The drawing under review shows one solid part. Ordinate dimensions are in mm from its lowest x, y, z. Coordinates: 2 decimals unless noted, no trailing zeros. Loops run counter-clockwise (first coordinate to the right, second up) from the corner with the lowest first, then second, coordinate; pieces in that order, holes last. Notation, with made-up numbers: M 69.5,-16 L 97.5,-16 A30 ccw 97.5,6 Z; hole C -26.5,83 d3. An arc over 180 degrees is marked long. Use one line per item in the form item = value.
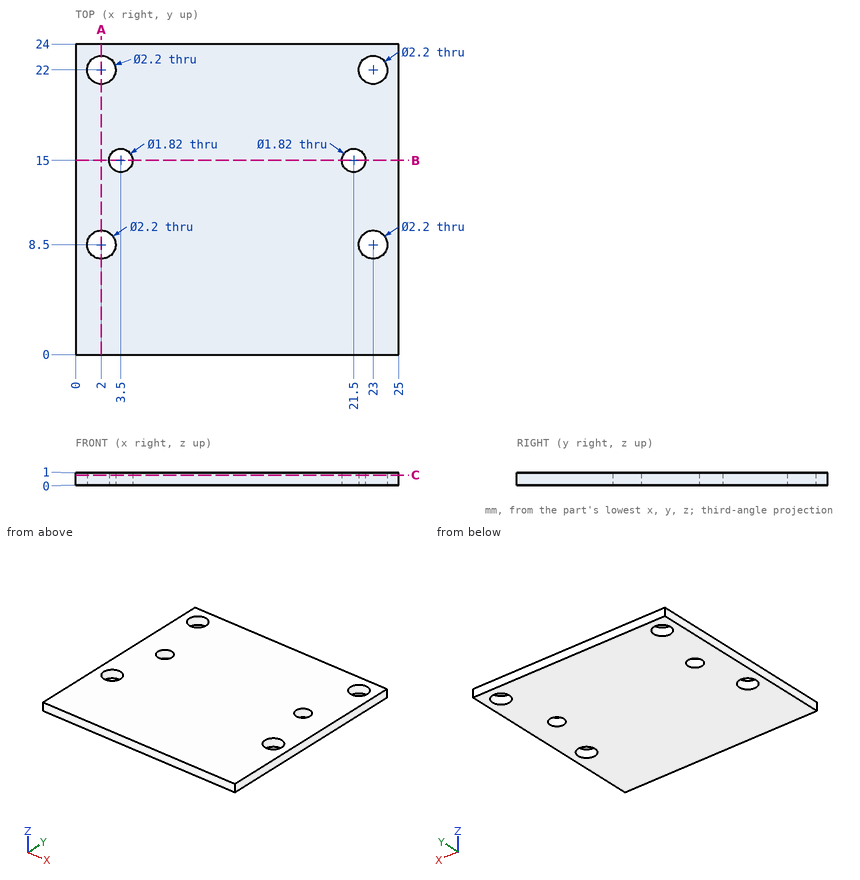
1. Consider section A-A on x = 2. Write out the cut boundary in (y, z), plus the area to 3 significant figures.
Computed values:
outline = M 0,0 L 7.4,0 L 7.4,1 L 0,1 Z; M 9.6,0 L 20.9,0 L 20.9,1 L 9.6,1 Z; M 23.1,0 L 24,0 L 24,1 L 23.1,1 Z
area = 19.6 mm2
2. Wall thickness on line 1 along X through (y, z) = (8.5, 0.7); line 2 along Y through (x, z) = (2, 0.7); line 3 along Y through (x, z) = (21.5, 0.45): over which ranges is each line inside the solid? List them lowest first. Write a range as from..to.
Computed values:
line_1 = 0..0.9, 3.1..21.9, 24.1..25
line_2 = 0..7.4, 9.6..20.9, 23.1..24
line_3 = 0..14.09, 15.91..24
3. Consider section B-B on y = 15. Write out the cut boundary in (x, z), plus the area to 3 significant figures.
Computed values:
outline = M 0,0 L 2.59,0 L 2.59,1 L 0,1 Z; M 4.41,0 L 20.59,0 L 20.59,1 L 4.41,1 Z; M 22.41,0 L 25,0 L 25,1 L 22.41,1 Z
area = 21.4 mm2
4. Consider section C-C on z = 0.8. Write out the cut boundary in (x, y).
Computed values:
outline = M 0,0 L 25,0 L 25,24 L 0,24 Z; hole C 2,8.5 d2.2; hole C 2,22 d2.2; hole C 3.5,15 d1.82; hole C 21.5,15 d1.82; hole C 23,8.5 d2.2; hole C 23,22 d2.2
5. For pin 1 Ø2 at (x, y) = (21.5, 15) entering from -Z; pin 2 Ø1.3 at (x, y) = (23, 8.5) entering from -Z, all flat-tipped, find the tip position at first contact; note any pin that passes through.
Computed values:
pin_1 = 0
pin_2 = through
